For this review, take the finished solid that the model builds, in its own axes (mm). Round coordinates to 2 decimals unless told otherwise and drop trailing zeros. Write each loop counter-clockwise with the first axis right and the second up, starting at its lowest first coordinate (ties: lowest second). Pieces come first, ordered by that corner, then holes. Notation, with made-up numbers: M 78.25,72.25 L 85.25,72.25 A19 cw 85.25,83.25 Z; hole C 46.5,72 d9. An arc over 180 degrees is marked long. Answer in a Markdown table with one row per item.
```python
from build123d import *

# Parameters (mm, degrees)
SKETCH1_W                = 6.5
SKETCH1_H                = 6.5
BOSS_EXTRUDE1_DEPTH      = 10
SKETCH2_W                = 5
SKETCH2_H                = 5
BOSS_EXTRUDE2_DEPTH      = 10.01
BOSS_EXTRUDE2_DEPTH_BACK = 0.01
SWEEP2_PROFILE_R         = 0.35
FILLET2_R                = 0.5


with BuildPart() as part:
    # Sketch1 → Boss-Extrude1 (new body)
    with BuildSketch(Plane(origin=(0, 0, 0), x_dir=(1, 0, 0), z_dir=(0, 1, 0))):
        Rectangle(SKETCH1_W, SKETCH1_H)
    boss_extrude1 = extrude(amount=BOSS_EXTRUDE1_DEPTH)

    # Sketch2 → Boss-Extrude2 (add, two sides)
    with BuildSketch(Plane(origin=(0, 0, 0), x_dir=(1, 0, 0), z_dir=(0, 1, 0))) as boss_extrude2_sk:
        Rectangle(SKETCH2_W, SKETCH2_H)
    extrude(amount=BOSS_EXTRUDE2_DEPTH)
    extrude(boss_extrude2_sk.sketch, amount=-BOSS_EXTRUDE2_DEPTH_BACK)

    # Sweep2: sweep along a path in Sketch4
    with BuildLine(Plane.XY) as sweep2_path:
        Line((3.2, 7.882896733), (3.25, 7.882896733))
        Line((3.25, 7.882896733), (3.75, 7.882896733))
        ThreePointArc((3.75, 7.882896733), (4.457106781, 7.590003514), (4.75, 6.882896733))
        Line((4.75, 6.882896733), (4.75, -68.117103267))
    # Sweep2 profile (on start of the path) → Sweep2 (sweep)
    with BuildSketch(Plane(origin=(3.2, 7.882896733, 0), x_dir=(0, 0, 1), z_dir=(1, 0, 0))):
        Circle(SWEEP2_PROFILE_R)
    sweep2 = sweep(path=sweep2_path.line)

    # Mirror1: Boss-Extrude1, Sweep2 across plane
    add(boss_extrude1.mirror(Plane(origin=(0, 0, 0), x_dir=(0, 0, 1), z_dir=(1, 0, 0))))
    add(sweep2.mirror(Plane(origin=(0, 0, 0), x_dir=(0, 0, 1), z_dir=(1, 0, 0))))

    # Fillet2
    fillet2_edges = [part.edges().sort_by_distance(p)[0] for p in [
        (3.25, 5, 3.25),
        (-3.25, 5, 3.25),
        (-3.25, 5, -3.25),
        (3.25, 5, -3.25),
    ]]
    fillet(fillet2_edges, radius=FILLET2_R)


solid = part.part
```
Q1. Insertion check: P1, Ø2, axis at x = 1, z = -2.5, coming from the -Y side; P2, Ø5, axis at x = 1.5, y = -40.5, coming from the +Z side. Each pin has a flat end and moves straight along its axis. Give the tip position at first contact, or say it passes through.
Found:
| item | result |
|---|---|
| P1 | y = -0.01 |
| P2 | through |
Q2. Take a section at C-C (y = -41). State the section outline as (x, z) points, then the cut area to 3 significant figures.
Found:
| item | result |
|---|---|
| outline | C -4.75,0 d0.7; C 4.75,0 d0.7 |
| area | 0.770 mm² |
Q3. For probe 1 along X at (y, z) = (-53.5, 0); probe 2 along Y at (x, z) = (-2.75, 1); probe 3 along Z at (x, y) = (4.5, -57.5), list the stretches that pass through material, from the lowest coordinate up.
Found:
| item | result |
|---|---|
| probe 1 | -5.1 to -4.4, 4.4 to 5.1 |
| probe 2 | 0 to 10 |
| probe 3 | -0.24 to 0.24 |
